Geometry: see drawing. Coordinates: mm, zero at the bounding-box minimum. A direction names the side the tool comes from. Give positions to 0.01 mm unless a question says otherwise; leave off trailing zeros. Write each loop counter-clockwise with the first axis right and the second up, starting at its lowest first coordinate (ties: lowest second). Pieces come first, ordered by that corner, then holes. Notation, with made-up numbers: M 60,-36.5 L 73,-36.5 A31 ccw 73,-11.5 Z; hole C -21,39 d10. An arc over 180 degrees is marked long. Use a Markdown table: item, result. Add a question column.
(1) Draft query along Y for the marked faces 3, 4 and 5. Return one class per face: released by +Y, released by -Y, zero draft, split by the parting line, or undercut.
(2) Material intervals for L1, parallel to X at y = 2.1, z = 3.25 (3 decimals); L2, parallel to Y at x = 4.5, z = 5.5; L3, parallel to X at y = 1.3, z = 3.25 (3 decimals), sorted ascending.
(3) Pin query (flat end, axial travel): pin 1 Ø1 at (y, z) = (2, 5.5) entering from +X; pin 2 Ø1.5 at (x, y) = (1.5, 1.5) entering from +Z. Return the tip coordinate at first contact, or that it passes through.
(4) Reachability of the marked faces 1 and 2 from +Z, -Z, +X, -X, +Y, -Y: full face, straight path, thin tool, end or side. Return the list, or none.
(5) Cut plane A-A (x = 6.25). Output: boundary loops of the cut face in (y, z).
(6) Cut plane D-D (x = 3.25). Output: boundary loops of the cut face in (y, z) (3 decimals).
(7) Cut plane B-B (z = 3.25). Output: boundary loops of the cut face in (x, y) (3 decimals).
(8) Cut plane C-C (y = 2.55). Output: boundary loops of the cut face in (x, z) (3 decimals), plus the area to 3 significant figures.
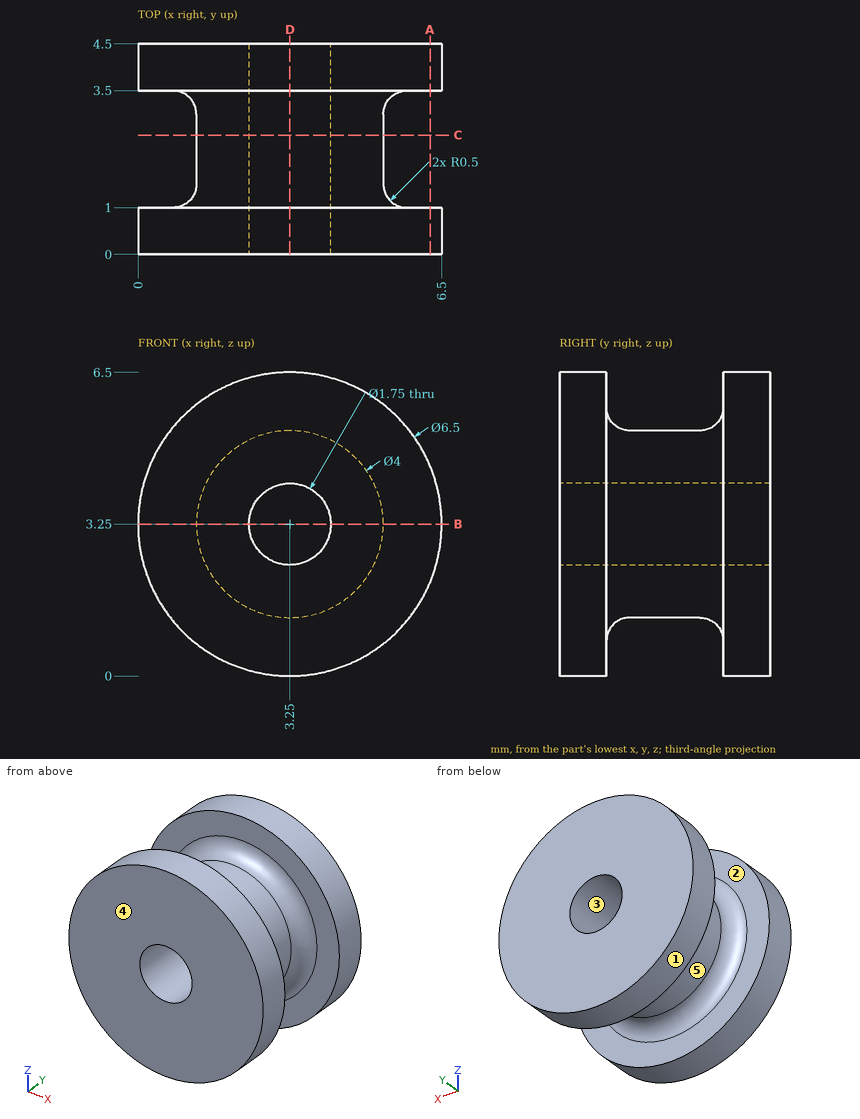
Answer list:
| question | item | result |
|---|---|---|
| 1 | face 3 | zero draft |
| 1 | face 4 | released by -Y |
| 1 | face 5 | undercut |
| 2 | L1 | 1.25 to 2.375, 4.125 to 5.25 |
| 2 | L2 | 0 to 1, 3.5 to 4.5 |
| 2 | L3 | 1.208 to 2.375, 4.125 to 5.292 |
| 3 | pin 1 | x = 4.22 |
| 3 | pin 2 | z = 6.27 |
| 4 | face 1 | +Y, -Y |
| 4 | face 2 | none |
| 5 | outline | M 0,2 L 1,2 L 1,4.5 L 0,4.5 Z; M 3.5,2 L 4.5,2 L 4.5,4.5 L 3.5,4.5 Z |
| 6 | outline | M 0,0 L 1,0 L 1,0.75 A0.5 cw 1.5,1.25 L 3,1.25 A0.5 cw 3.5,0.75 L 3.5,0 L 4.5,0 L 4.5,2.375 L 0,2.375 Z; M 0,4.125 L 4.5,4.125 L 4.5,6.5 L 3.5,6.5 L 3.5,5.75 A0.5 cw 3,5.25 L 1.5,5.25 A0.5 cw 1,5.75 L 1,6.5 L 0,6.5 Z |
| 7 | outline | M 0,0 L 2.375,0 L 2.375,4.5 L 0,4.5 L 0,3.5 L 0.75,3.5 A0.5 cw 1.25,3 L 1.25,1.5 A0.5 cw 0.75,1 L 0,1 Z; M 4.125,0 L 6.5,0 L 6.5,1 L 5.75,1 A0.5 cw 5.25,1.5 L 5.25,3 A0.5 cw 5.75,3.5 L 6.5,3.5 L 6.5,4.5 L 4.125,4.5 Z |
| 8 | outline | C 3.25,3.25 d4; hole C 3.25,3.25 d1.75 |
| 8 | area | 10.2 mm² |
